```python
from build123d import *

# Parameters (mm, degrees)
SKETCH1_W                 = 65.44
SKETCH1_H                 = 122
BOSS_EXTRUDE1_DEPTH       = 6.35
M4X0_7_TAPPED_HOLE1_D     = 3.3
M4X0_7_TAPPED_HOLE1_DEPTH = 6.35
M8_CLEARANCE_HOLE1_D      = 9
M8_CLEARANCE_HOLE1_DEPTH  = 6.35
CUT_EXTRUDE2_REACH        = 8.35
SKETCH14_R                = 12.5


with BuildPart() as part:
    # Sketch1 → Boss-Extrude1 (new body)
    with BuildSketch(Plane.XY):
        Rectangle(SKETCH1_W, SKETCH1_H)
    extrude(amount=BOSS_EXTRUDE1_DEPTH)

    # M4x0.7 Tapped Hole1
    with Locations(Plane.XY.offset(6.35)):
        with Locations((0, 25), (-21.650635095, 12.5), (-21.650635095, -12.5), (0, -25), (21.650635095, -12.5), (21.650635095, 12.5)):
            Hole(M4X0_7_TAPPED_HOLE1_D / 2, depth=M4X0_7_TAPPED_HOLE1_DEPTH)

    # M8 Clearance Hole1
    with Locations(Plane.XY.offset(6.35)):
        with Locations((-15.37, 53), (15.37, 53), (15.37, -53), (-15.37, -53)):
            Hole(M8_CLEARANCE_HOLE1_D / 2, depth=M8_CLEARANCE_HOLE1_DEPTH)

    # Sketch14 → Cut-Extrude2 (cut, up to next)
    with BuildSketch(Plane.XY.offset(6.35), mode=Mode.PRIVATE) as cut_extrude2_sk1:
        Circle(SKETCH14_R)
    cut_extrude2_tool1 = extrude(cut_extrude2_sk1.sketch, amount=-CUT_EXTRUDE2_REACH, mode=Mode.PRIVATE) & part.part
    add(cut_extrude2_tool1.solids().sort_by_distance((0, 0, 6.35))[0], mode=Mode.SUBTRACT)


solid = part.part
```
Read the model definition and answer for the solid it produces. Units are mm, in the model's axes. Coordinates: 2 decimals unless noted, no trailing zeros. Loops run counter-clockwise (first coordinate to the right, second up) from the corner with the lowest first, then second, coordinate; pieces in that order, holes last. Notation, with made-up numbers: (-39.5, -19) -> (-32.5, -19) arc R15 ccw to (-32.5, -10) -> close; hole circle Ø7 at (-24.5, -13). An arc over 180 degrees is marked (long way). Return JSON: item names as keys, results as strings.
Item 1: Find the intervals of material crossed by probe 1 along Y at (x, z) = (-15.37, 5.25); probe 2 along X at (y, z) = (-54.5, 2); probe 3 along Y at (x, z) = (0, 0.75), in increasing order.
Answers:
{"probe 1": "y = -61 to -57.5, -48.5 to 48.5, 57.5 to 61", "probe 2": "x = -32.72 to -19.61, -11.13 to 11.13, 19.61 to 32.72", "probe 3": "y = -61 to -26.65, -23.35 to -12.5, 12.5 to 23.35, 26.65 to 61"}
Item 2: Find section B-B (z = 1.75). Count the separate pieces of the cut face and the enclosed holes in it, plus the area to 3 significant figures.
Answers:
{"separate pieces": "1", "enclosed holes": "11", "area": "7,190 mm2"}
Item 3: Find section D-D (y = -53). Determine the outline of the cut face in (x, z).
Answers:
{"outline": "(-32.72, 0) -> (-19.87, 0) -> (-19.87, 6.35) -> (-32.72, 6.35) -> close; (-10.87, 0) -> (10.87, 0) -> (10.87, 6.35) -> (-10.87, 6.35) -> close; (19.87, 0) -> (32.72, 0) -> (32.72, 6.35) -> (19.87, 6.35) -> close"}
Item 4: Find section A-A (x = 0). Determine the outline of the cut face in (y, z), plus the area to 3 significant figures.
Answers:
{"outline": "(-61, 0) -> (-26.65, 0) -> (-26.65, 6.35) -> (-61, 6.35) -> close; (-23.35, 0) -> (-12.5, 0) -> (-12.5, 6.35) -> (-23.35, 6.35) -> close; (12.5, 0) -> (23.35, 0) -> (23.35, 6.35) -> (12.5, 6.35) -> close; (26.65, 0) -> (61, 0) -> (61, 6.35) -> (26.65, 6.35) -> close", "area": "574 mm2"}
Item 5: Find section C-C (y = 25). Determine the outline of the cut face in (x, z).
Answers:
{"outline": "(-32.72, 0) -> (-1.65, 0) -> (-1.65, 6.35) -> (-32.72, 6.35) -> close; (1.65, 0) -> (32.72, 0) -> (32.72, 6.35) -> (1.65, 6.35) -> close"}
Item 6: For a pull along X with two mould halves and no side action, classify faces 1 (the flat face through (0, -61, 3)), 2 (the cylindrical face through (0.215, -23.364, 3.131)), 3 (the flat face through (32.72, -1, 3)) as +X half, -X half, draft (parallel to the pull), parting line (faces both ways), or undercut.
Answers:
{"face 1": "draft", "face 2": "undercut", "face 3": "+X half"}
Item 7: Flat-ended cylindrical pins translate along their axes: P1, Ø10, axis at x = -8, y = 33.5, coming from the -Z side; P2, Ø2.5, axis at x = 21.65, y = -12.5, coming from the -Z side. Find the tip coordinate at first contact, or state that the pin passes through.
Answers:
{"P1": "stops at z = 0", "P2": "passes through"}
